Autodesk Inventor part; units mm, degrees
ref_plane "Work Plane1" through (0, 0, 43.815) normal (0, 0, 1) x (1, 0, 0)
ref_plane "YZ Plane" through (0, 0, 0) normal (1, 0, 0) x (0, 1, 0)
ref_plane "XZ Plane" through (0, 0, 0) normal (0, 1, 0) x (-1, 0, 0)
sketch "Sketch1" plane through (0, 0, 0) normal (0, 0, 1) x (1, 0, 0)
  line L0 (0, 0) -> (112.268, 0)
  line L1 (112.268, 0) -> (112.268, 67.31)
  line L2 (112.268, 67.31) -> (0, 67.31)
  line L3 (0, 67.31) -> (0, 0)
  dimension "d0" = 112.268
  dimension "d1" = 67.31
extrude "Extrusion1" add sketch "Sketch1" along normal blind 87.63
shell "Shell1" thickness 3.81 removed faces 1 at (74.8453, 67.31, 29.21)
sketch "Sketch2" plane through (0, 0, 87.63) normal (0, 0, 1) x (1, 0, 0)
  line L0 (112.268, 67.31) -> (0, 67.31)
  line L1 (0, 0) -> (112.268, 0)
  line L2 (10.414, 67.31) -> (15.494, 67.31)
  line L3 (15.494, 67.31) -> (15.494, 0)
  line L4 (15.494, 0) -> (10.414, 0)
  line L5 (10.414, 0) -> (10.414, 67.31)
  line L6 (25.654, 0) -> (30.734, 0)
  line L7 (30.734, 0) -> (30.734, 67.31)
  line L8 (30.734, 67.31) -> (25.654, 67.31)
  line L9 (25.654, 67.31) -> (25.654, 0)
  line L10 (86.614, 67.31) -> (81.534, 67.31)
  line L11 (81.534, 67.31) -> (81.534, 0)
  line L12 (81.534, 0) -> (86.614, 0)
  line L13 (86.614, 0) -> (86.614, 67.31)
  line L14 (96.774, 0) -> (101.854, 0)
  line L15 (101.854, 0) -> (101.854, 67.31)
  line L16 (101.854, 67.31) -> (96.774, 67.31)
  line L17 (96.774, 67.31) -> (96.774, 0)
  point P0 (56.134, 0)
  dimension "d5" = 5.08
  dimension "d6" = 5.08
  dimension "d7" = 5.08
  dimension "d8" = 5.08
  dimension "d9" = 10.16
  dimension "d10" = 10.16
  dimension "d11" = 50.8
  dimension "d12" = 25.4
extrude "Extrusion2" add sketch "Sketch2" along normal blind 2.54 contours L15 L1 L17 L0 | L13 L1 L11 L0 | L7 L1 L9 L0 | L3 L1 L5 L0
ref_plane "Work Plane1" through (0, 0, 43.815) normal (0, 0, 1) x (1, 0, 0)
mirror "Mirror1" about plane through (0, 0, 43.815) normal (0, 0, 1) of "Extrusion2"
fillet "Fillet1" radius 2.54 12 edges at (12.954, 0, 90.17) (28.194, 0, 90.17) (20.574, 0, 87.63) (84.074, 0, 90.17) (91.694, 0, 87.63) (99.314, 0, 90.17) (12.954, 0, -2.54) (20.574, 0, 0) (28.194, 0, -2.54) (91.694, 0, 0) (99.314, 0, -2.54) (84.074, 0, -2.54)
sketch "Sketch3" plane through (0, 0, 87.63) normal (0, 0, 1) x (1, 0, 0)
  line L0 (65.8267, 5.2092) -> (47.5136, 5.3082)
  line L1 (47.5136, 5.3082) -> (38.4421, 21.2186)
  line L2 (38.4421, 21.2186) -> (47.6874, 37.0338)
  line L3 (47.6874, 37.0338) -> (65.9845, 37.0338)
  line L4 (65.9845, 37.0338) -> (75.1503, 21.1582)
  line L5 (75.1503, 21.1582) -> (65.8267, 5.2092)
  line L6 (50.3144, 32.4551) -> (43.729, 21.19)
  line L7 (43.729, 21.19) -> (50.1818, 9.8726)
  line L8 (50.1818, 9.8726) -> (63.208, 9.8021)
  line L9 (63.208, 9.8021) -> (69.855, 21.1725)
  line L10 (69.855, 21.1725) -> (63.341, 32.4551)
  line L11 (63.341, 32.4551) -> (50.3144, 32.4551)
  line L12 (38.5123, 28.5967) -> (38.5123, 46.9115)
  line L13 (38.5123, 46.9115) -> (43.091, 46.9115)
  line L14 (43.091, 46.9115) -> (43.091, 36.4292)
  line L15 (43.091, 36.4292) -> (38.5123, 28.5967)
  line L16 (47.6697, 59.0116) -> (52.2484, 59.0116)
  line L17 (52.2484, 59.0116) -> (52.2484, 40.6967)
  line L18 (65.9845, 40.6967) -> (65.9845, 59.0116)
  line L19 (65.9845, 59.0116) -> (61.4058, 59.0116)
  line L20 (61.4058, 59.0116) -> (61.4058, 40.6967)
  line L21 (75.1419, 28.4986) -> (75.1419, 46.9115)
  line L22 (75.1419, 46.9115) -> (70.5632, 46.9115)
  line L23 (70.5632, 46.9115) -> (70.5632, 36.4292)
  line L24 (70.5632, 36.4292) -> (75.1419, 28.4986)
  line L25 (54.5377, 63.5903) -> (54.5377, 40.6967)
  line L26 (54.5377, 40.6967) -> (59.1164, 40.6967)
  line L27 (59.1164, 40.6967) -> (59.1164, 63.5903)
  line L28 (59.1164, 63.5903) -> (54.5377, 63.5903)
  line L29 (61.4058, 40.6967) -> (65.9845, 40.6967)
  line L30 (52.2484, 59.0116) -> (54.5377, 59.0116) construction
  line L31 (61.4058, 59.0116) -> (59.1164, 59.0116) construction
  line L32 (47.6697, 59.0116) -> (47.6697, 40.6967)
  line L33 (47.6697, 40.6967) -> (52.2484, 40.6967)
  line L34 (81.534, 67.31) -> (81.534, 2.54)
  point P0 (0, 0)
  point P1 (56.3847, 20.5734)
  point P2 (56.6949, 9.8373)
  dimension "d16" = 18.3134
  dimension "d17" = 4.5787
  dimension "d18" = 3.663
  dimension "d19" = 3.663
  dimension "d20" = 4.5787
  dimension "d21" = 4.5787
  dimension "d22" = 4.5787
  dimension "d23" = 4.5787
  dimension "d24" = 3.663
  dimension "d25" = 18.3148
  dimension "d26" = 18.3148
  dimension "d27" = 22.8935
  dimension "d28" = 4.5787
  dimension "d29" = 4.5787
  dimension "d30" = 4.5787
  dimension "d31" = 2.2894
  dimension "d32" = -4.5964
  dimension "d33" = 24.8391
extrude "Extrusion3" add sketch "Sketch3" along normal blind 2.54
fillet "Fillet2" radius 2.54 4 edges at (0, 33.655, 87.63) (112.268, 33.655, 87.63) (112.268, 33.655, 0) (0, 33.655, 0)
equation "\"d5\" = d6"
equation "\"d7\" = d6"
equation "\"d8\" = d7"
equation "\"d10\" = d9"
properties part number "Janus wire holder"
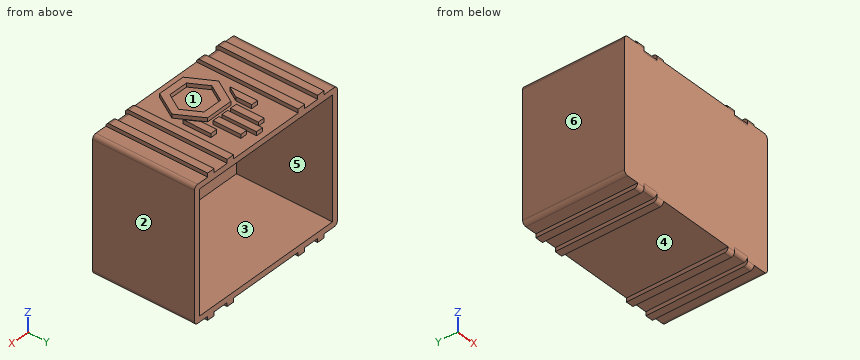
Part model, mm, in its own coordinate system. Face numbers are marked on the shaded views. A direction names the side the tool comes from. Round coordinates to 2 decimals unless told otherwise and drop trailing zeros. Loops run counter-clockwise (first coordinate to the right, second up) from the corner with the lowest first, then second, coordinate; pieces in that order, holes last. Notation, with made-up numbers: (17.5, 82.25) -> (72.5, 82.25) arc R20 cw to (72.5, 118.25) -> close; hole circle Ø4 at (-35, 2.5). An arc over 180 degrees is marked (long way). Use a Markdown table: item, result.
1) Tool access for the marked faces 5 and 6: list every direction of +Z, -Z, +X, -X, +Y, -Y with a clear straight run to the whole face (end or side of a thin tool).
The answers:
| item | result |
|---|---|
| face 5 | +Y |
| face 6 | +Z, -Z, -X, +Y, -Y |
2) Pull direction Z, two halves, no side cores. Call the marked faces 1, 2, 3 and 4: pulls with the +Z half, pulls with the -Z half, needs draft (parallel to the pull), parting line crosses it, or undercut.
The answers:
| item | result |
|---|---|
| face 1 | pulls with the +Z half |
| face 2 | needs draft |
| face 3 | undercut |
| face 4 | pulls with the -Z half |
3) Drop flat-ended pins along their axis: pin 1 Ø1 at (x, y) = (93, 44) entering from +Z; pin 2 Ø2 at (x, z) = (50.5, 89) entering from -Y; pin 3 Ø0.8 at (y, z) = (23, -1.5) entering from -X. Give the stop position or say it passes through.
The answers:
| item | result |
|---|---|
| pin 1 | stops at z = 87.63 |
| pin 2 | stops at y = 5.29 |
| pin 3 | stops at x = 10.41 |
4) Cut at C-C, the plane x = 45.5. List the corners of the cut face in (y, z), and give its area (3 significant figures).
The answers:
| item | result |
|---|---|
| outline | (0, 0) -> (67.31, 0) -> (67.31, 3.81) -> (3.81, 3.81) -> (3.81, 83.82) -> (67.31, 83.82) -> (67.31, 87.63) -> (33.29, 87.63) -> (33.29, 90.17) -> (24.22, 90.17) -> (24.22, 87.63) -> (18.08, 87.63) -> (18.08, 90.17) -> (8.84, 90.17) -> (8.84, 87.63) -> (0, 87.63) -> close |
| area | 864 mm2 |
5) Probe line 1 (Z direction, x = 26.5, y = 7.5); line 2 (Z direction, x = 81, y = 58); line 3 (X direction, y = 60.5, z = 21.5). List the from-to ranges inside material, lowest first. Write a range as [from, to].
The answers:
| item | result |
|---|---|
| line 1 | z = [-2.54, 3.81], [83.82, 90.17] |
| line 2 | z = [0, 3.81], [83.82, 87.63] |
| line 3 | x = [0, 3.81], [108.46, 112.27] |
6) Cut at A-A, the plane z = 40.5. List the corners of the cut face in (x, y), and give its area (3 significant figures).
The answers:
| item | result |
|---|---|
| outline | (0, 0) -> (112.27, 0) -> (112.27, 67.31) -> (108.46, 67.31) -> (108.46, 3.81) -> (3.81, 3.81) -> (3.81, 67.31) -> (0, 67.31) -> close |
| area | 912 mm2 |
7) Cut at B-B, the plane x = 85. List the corners of the cut face in (y, z), and give its area (3 significant figures).
The answers:
| item | result |
|---|---|
| outline | (0, 0) arc R2.54 ccw to (2.54, -2.54) -> (67.31, -2.54) -> (67.31, 3.81) -> (3.81, 3.81) -> (3.81, 83.82) -> (67.31, 83.82) -> (67.31, 90.17) -> (2.54, 90.17) arc R2.54 ccw to (0, 87.63) -> close |
| area | 1,160 mm2 |
